Could you check a few things on this model? Use its own coordinates, in mm. Face numbers are marked on the shaded views. A direction names the side the tool comes from. Coordinates: 2 decimals unless noted, no trailing zeros. Order: outer loops, then holes, each group sorted by start corner. A loop starts at its lowest first (then second) coordinate and runs counter-clockwise, first axis right, second up. Notation, with made-up numbers: M 42,24 L 87,24 A14 cw 87,28 Z; hole C -26,53 d3. An arc over 180 degrees is marked long. One line per question, with ' | ' between items. Start each with the question number.
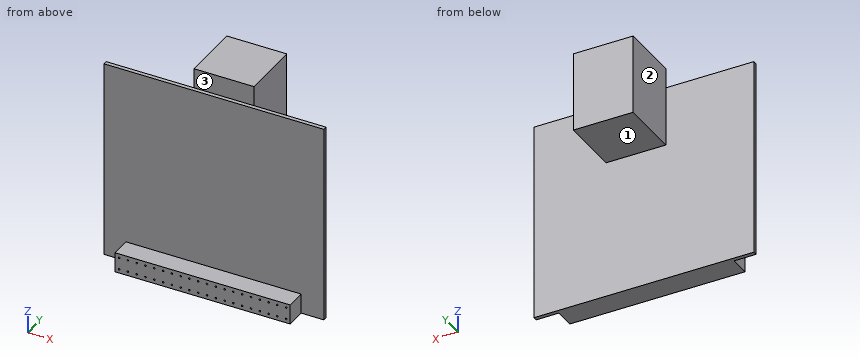
from build123d import *

# Parameters (mm, degrees)
SKETCH_1_W                  = 55
SKETCH_1_H                  = 50
EXTRUDE_1_DEPTH             = 1
SKETCH_2_W                  = 15
SKETCH_2_H                  = 20
EXTRUDE_2_DEPTH             = 15
SKETCH_11_W                 = 43.8
SKETCH_11_H                 = 5
EXTRUDE_7_DEPTH             = 5
SKETCH_12_R                 = 0.2
CUT_EXTRUDE_1_DEPTH         = 5
PATTERN_LINEAR_1_COUNT      = 20
PATTERN_LINEAR_1_PITCH      = 2.2
PATTERN_LINEAR_1_COUNT_DIR2 = 2
PATTERN_LINEAR_1_PITCH_DIR2 = 3


with BuildPart() as part:
    # 草图1 → 凸台-拉伸1 (new body)
    with BuildSketch(Plane(origin=(0, 0, 0), x_dir=(1, 0, 0), z_dir=(0, 1, 0))):
        with Locations((-0.456810631, -5.722591362)):
            Rectangle(SKETCH_1_W, SKETCH_1_H)
    extrude(amount=EXTRUDE_1_DEPTH)

    # 草图2 → 凸台-拉伸2 (add)
    with BuildSketch(Plane(origin=(0, 1, 0), x_dir=(1, 0, 0), z_dir=(0, 1, 0))):
        with Locations((1.543189369, -25.722591362)):
            Rectangle(SKETCH_2_W, SKETCH_2_H)
    extrude(amount=EXTRUDE_2_DEPTH)

    # 草图11 → 凸台-拉伸7 (add)
    with BuildSketch(Plane(origin=(0, 0, 0), x_dir=(-1, 0, 0), z_dir=(0, -1, 0))):
        with Locations((0.551477247, 16.777408638)):
            Rectangle(SKETCH_11_W, SKETCH_11_H)
    extrude(amount=EXTRUDE_7_DEPTH)

    # 草图12 → 切除-拉伸1 (cut)
    with BuildSketch(Plane(origin=(0, -5, 0), x_dir=(-1, 0, 0), z_dir=(0, -1, 0))):
        with Locations(Location((21.451477247, 15.277408638, 0), (0, 0, 90))):
            Circle(SKETCH_12_R)
    cut_extrude_1 = extrude(amount=-CUT_EXTRUDE_1_DEPTH, mode=Mode.SUBTRACT)

    # 阵列(线性)1: Cut-Extrude 1 20 × 2
    with Locations(*[(i * PATTERN_LINEAR_1_PITCH, 0, -j * PATTERN_LINEAR_1_PITCH_DIR2) for i in range(PATTERN_LINEAR_1_COUNT) for j in range(PATTERN_LINEAR_1_COUNT_DIR2) if (i, j) != (0, 0)]):
        add(cut_extrude_1, mode=Mode.SUBTRACT)


solid = part.part
(1) Imagine slicing it at A-A, the plane z = 17. Write out the boundary of the cut face in (x, y), plus the area to 3 significant figures.
(2) Imagine slicing it at B-B, the plane y = 3. Write out the boundary of the cut face in (x, z), plus the area to 3 significant figures.
(3) For P1, Ø6, axis at y = 9.5, z = 23.5, coming from the +X side; P2, Ø2, axis at x = 12.5, z = 9, coming from the -Y side; P3, Ø1.5, axis at y = 8, z = 22, coming from the -X side, each with a flat end and sliding along its axis, tell me the tip position at first contact or that it passes through.
(4) If I drill on line 1 along Z through (x, y) = (-17, -1.75); line 2 along Y through (x, z) = (1, -15.5); line 3 along Z through (x, y) = (7, -1.5), over which ranges is the centre line in solid material (lowest first)? Write a range as from..to.
(5) Imagine slicing it at D-D, the plane z = -6.5. Write out the boundary of the cut face in (x, y), plus the area to 3 significant figures.
(6) On a 3-axis mill with a long thin cutter (end or side, diameter ignored), from which of +Z, -Z, +X, -X, +Y, -Y can I reach the whole of each face in a straight line? I mean the marked faces 1, 2 and 3. Say none if no direction works.
(7) Imagine slicing it at C-C, the plane y = -2. Count the separate pieces of the cut face and the enclosed holes in it, plus the area to 3 significant figures.
Answers:
1) outline: M -27.96,0 L 27.04,0 L 27.04,1 L 9.04,1 L 9.04,16 L -5.96,16 L -5.96,1 L -27.96,1 Z | area: 280 mm²
2) outline: M -5.96,15.72 L 9.04,15.72 L 9.04,35.72 L -5.96,35.72 Z | area: 300 mm²
3) P1: x = 9.04 | P2: y = 0 | P3: x = -5.96
4) line 1: -19.28..-18.47, -18.08..-15.47, -15.08..-14.28 | line 2: -5..1 | line 3: -19.28..-18.41, -18.14..-15.41, -15.14..-14.28
5) outline: M -27.96,0 L 27.04,0 L 27.04,1 L -27.96,1 Z | area: 55.0 mm²
6) face 1: -Z, +X, -X, +Y | face 2: +Z, -Z, -X, +Y | face 3: +Z, +X, -X, -Y
7) separate pieces: 1 | enclosed holes: 40 | area: 214 mm²
